Could you check a few things on this model? Use its own coordinates, in mm. Round coordinates to 2 decimals unless told otherwise and drop trailing zeros. Order: outer loops, then holes, each group sorted by start corner. A loop starts at its lowest first (then second) coordinate and runs counter-clockwise, first axis right, second up. Notation, with made-up numbers: (41, -10.5) - (66, -10.5) arc R17 ccw to (66, 16.5) - close; hole circle Ø10 at (76.25, 31.5). An arc over 180 degrees is marked (long way). Return JSON: item names as keys, results as strings. Group by question number.
from build123d import *

# Parameters (mm, degrees)
F1_DEPTH = 6.35


with BuildPart() as f1:
    # F0 (on Top) → F1 (new body)
    with BuildSketch(Plane.XY):
        Polygon((0, -76.2), (0, 0), (-76.2, 0), (-76.2, -38.1), (-38.1, -76.2), align=None)
        Polygon((0, 76.2), (0, 0), (76.2, 0), (76.2, 38.1), (38.1, 76.2), align=None)
        Polygon((-76.2, 0), (0, 0), (0, 76.2), (-38.1, 76.2), (-76.2, 38.1), align=None)
        Polygon((76.2, 0), (0, 0), (0, -76.2), (38.1, -76.2), (76.2, -38.1), align=None)
    extrude(amount=F1_DEPTH)


solid = f1.part
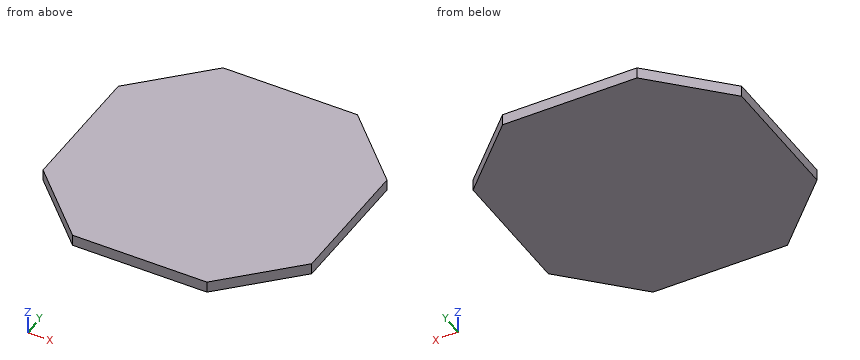
1) I want a section at B-B, the plane y = -60. List the corners of the cut face in (x, z) for me.
2) If I drill on line 1 along X through (y, z) = (54, 5); line 2 along Y through (x, z) = (-70, 5.75); line 3 along X through (y, z) = (-46.5, 3.5), over which ranges is the centre line in solid material (lowest first)? Write a range as from..to.
3) I want a section at C-C, the plane x = 50.5. List the corners of the cut face in (y, z) for me, plus the area to 3 significant figures.
4) I want a section at A-A, the plane z = 2.5. List the corners of the cut face in (x, y) for me, plus the area to 3 significant figures.
5) Will these pins go through, and if not, where does the flat tip stop? pin 1 (5 mm diameter, centred on x = 48, y = 18.5, fed in from -Z); pin 2 (3 mm diameter, centred on x = -44.5, z = 1, fed in from +Y).
Outcome:
{
 "1": {"outline": "(-54.3, 0) - (54.3, 0) - (54.3, 6.35) - (-54.3, 6.35) - close"},
 "2": {"line 1": "-60.3..60.3", "line 2": "-44.3..44.3", "line 3": "-67.8..67.8"},
 "3": {"outline": "(-63.8, 0) - (63.8, 0) - (63.8, 6.35) - (-63.8, 6.35) - close", "area": "810 mm^2"},
 "4": {"outline": "(-76.2, -38.1) - (-38.1, -76.2) - (38.1, -76.2) - (76.2, -38.1) - (76.2, 38.1) - (38.1, 76.2) - (-38.1, 76.2) - (-76.2, 38.1) - close", "area": "20,300 mm^2"},
 "5": {"pin 1": "z = 0", "pin 2": "y = 71.3"}
}
